Job drawing, mm, ordinate dimensions from the low corner. One solid piece. Coordinates: 2 decimals unless noted, no trailing zeros. Loops run counter-clockwise (first coordinate to the right, second up) from the corner with the lowest first, then second, coordinate; pieces in that order, holes last. Notation, with made-up numbers: M 62.5,-39.5 L 100.5,-39.5 A10 cw 100.5,-29.5 Z; hole C 66,-23.75 d3. An arc over 180 degrees is marked long. Write each question's results on one line, items separated by ' | '. Start each with the question number.
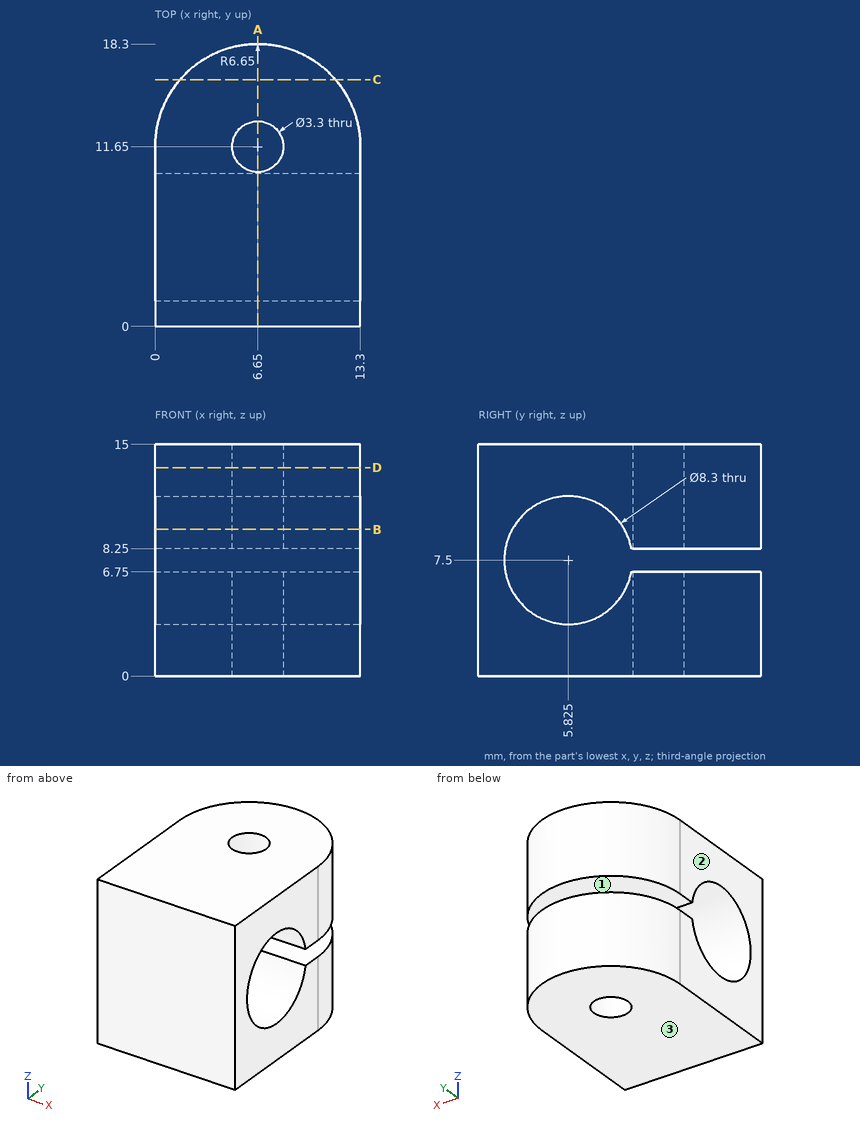
1. Pin check, flat tips, straight feed: pin 1 (2 mm diameter, centred on y = 15.5, z = 12.5, fed in from +X); pin 2 (6 mm diameter, centred on y = 7, z = 10, fed in from -X). Stop position of each tip, or through.
2. Band-saw the part on D-D, the plane z = 13.5. List the corners of the cut face in (x, y).
3. Band-saw the part on C-C, the plane y = 16. List the corners of the cut face in (x, z).
4. Mould opens along Z. For the marked faces 1, 2 and 3 say: +Z half, -Z half, draft (parallel to the pull), parting line (faces both ways), or undercut.
5. Wall check: line 1 along Z through (x, y) = (8.5, 11.25); line 2 along Y through (x, z) = (6.65, 13.75); line 3 along Y through (x, z) = (5.5, 8.5). Give the ranges that are in metal, low to high.
6. Band-saw the part on A-A, the plane x = 6.65. List the corners of the cut face in (y, z) (3 decimals), plus the area to 3 significant figures.
7. Band-saw the part on B-B, the plane z = 9.5. List the corners of the cut face in (x, y).
Checked values:
1) pin 1: x = 12.66 | pin 2: x = 0
2) outline: M 0,0 L 13.3,0 L 13.3,11.65 A6.65 ccw 0,11.65 Z; hole C 6.65,11.65 d3.3
3) outline: M 1.62,0 L 11.68,0 L 11.68,6.75 L 1.62,6.75 Z; M 1.62,8.25 L 11.68,8.25 L 11.68,15 L 1.62,15 Z
4) face 1: undercut | face 2: draft | face 3: -Z half
5) line 1: 0 to 6.75, 8.25 to 15 | line 2: 0 to 10, 13.3 to 18.3 | line 3: 0 to 1.8, 9.85 to 10.47, 12.83 to 18.2
6) outline: M 0,0 L 10,0 L 10,6.75 L 9.907,6.75 A4.15 cw long 9.907,8.25 L 10,8.25 L 10,15 L 0,15 Z; M 13.3,0 L 18.3,0 L 18.3,6.75 L 13.3,6.75 Z; M 13.3,8.25 L 18.3,8.25 L 18.3,15 L 13.3,15 Z | area: 163 mm²
7) outline: M 0,0 L 13.3,0 L 13.3,2.19 L 0,2.19 Z; M 0,9.46 L 13.3,9.46 L 13.3,11.65 A6.65 ccw 0,11.65 Z; hole C 6.65,11.65 d3.3
